Source: CAD feature listing. Evaluate the final solid. Frame: model axes, mm. A direction names the side the tool comes from. Give positions to 0.01 mm unless a question says otherwise; leave off trailing zeros. Order: outer loops, then holes, each group sorted by start corner. A loop starts at its lowest first (then second) coordinate and runs counter-clockwise, first axis right, second up. Notation, with made-up numbers: M 62,34 L 87,34 A9 ccw 87,43 Z; hole C -32,37.5 d10. An arc over 180 degrees is marked long. Answer in a Markdown table with one row per item. Add a question column.
(1) Pin query (flat end, axial travel): P1, Ø1.5, axis at x = -9, y = 8.5, coming from the -Z side; P2, Ø2, axis at y = 17.5, z = -16.5, coming from the -X side; P3, Ø1, axis at y = 12.5, z = -17.5, coming from the +X side. Return the tip coordinate at first contact, or that it passes through.
(2) Mould query, pull axis X, two halves, no side actions, for faces 4 (the face through (-25, 10, -30)), 5 (the face through (-20, 20, -5)), 6 (the face through (-22, 9.86, -24.54)). Classes: pulls with the +X half, pulls with the -X half, needs draft (parallel to the pull), parting line crosses it, or undercut.
(3) Section query C-C, the plane y = 8.5. Return loops of the section in (x, z).
(4) Section query A-A, the plane z = -9. Return loops of the section in (x, y).
(5) Section query D-D, the plane y = 18.5. Return loops of the section in (x, z), plus the area to 3 significant figures.
(6) Section query B-B, the plane x = -5. Return loops of the section in (y, z).
(7) Set-up query: faces 1 (the face through (-7.2, 9.9, -15)), 2 (the face through (-47.2, 9.9, -15)), 3 (the face through (-20, 0, -5)). Return all of +Z, -Z, +X, -X, +Y, -Y with unobstructed straight access to the full face (end or side cutting, diameter ignored); none if empty.
(8) Material intervals for line 1 along Y through (x, z) = (-5, -9.5); line 2 along Z through (x, y) = (-20.5, 18.75); line 3 along Z through (x, y) = (-5, 4), sorted ascending.
from build123d import *

# Parameters (mm, degrees)
BOSS_EXTRUDE1_DEPTH = 20
SKETCH3_R           = 10
CUT_EXTRUDE1_DEPTH  = 62.64414003
SKETCH4_R           = 2
CUT_EXTRUDE2_DEPTH  = 56.901699437


with BuildPart() as part:
    # Sketch2 → Boss-Extrude1 (new body)
    with BuildSketch(Plane(origin=(0, 0, 0), x_dir=(1, 0, 0), z_dir=(0, 1, 0))):
        with BuildLine():
            Line((-50, 0), (0, 0))
            Line((0, 0), (0, 15))
            Line((0, 15), (-10, 15))
            ThreePointArc((-10, 15), (-25, 30), (-40, 15))
            Line((-40, 15), (-50, 15))
            Line((-50, 15), (-50, 0))
        make_face()
    extrude(amount=BOSS_EXTRUDE1_DEPTH)

    # Sketch3 → Cut-Extrude1 (cut, through all)
    with BuildSketch(Plane(origin=(0, 0, 0), x_dir=(-1, 0, 0), z_dir=(0, -1, 0))):
        with Locations(Location((25, 15, 0), (0, 0, 90))):
            Circle(SKETCH3_R)
    extrude(amount=-CUT_EXTRUDE1_DEPTH, mode=Mode.SUBTRACT)

    # Sketch4 → Cut-Extrude2 (cut, through all)
    with BuildSketch(Plane(origin=(0, 0, -15), x_dir=(-1, 0, 0), z_dir=(0, 0, -1))):
        with Locations((45, 10)):
            Circle(SKETCH4_R)
        with Locations((5, 10)):
            Circle(SKETCH4_R)
    extrude(amount=-CUT_EXTRUDE2_DEPTH, mode=Mode.SUBTRACT)


solid = part.part
Values follow:
| question | item | result |
|---|---|---|
| 1 | P1 | stops at z = -15 |
| 1 | P2 | stops at x = -39.99 |
| 1 | P3 | stops at x = -10.13 |
| 2 | face 4 | parting line crosses it |
| 2 | face 5 | needs draft |
| 2 | face 6 | undercut |
| 3 | outline | M -50,-15 L -46.32,-15 L -46.32,0 L -50,0 Z; M -43.68,-15 L -40,-15 A15 ccw -10,-15 L -6.32,-15 L -6.32,0 L -43.68,0 Z; M -3.68,-15 L 0,-15 L 0,0 L -3.68,0 Z; hole C -25,-15 d20 |
| 4 | outline | M -50,0 L -33,0 L -33,20 L -50,20 Z; M -17,0 L 0,0 L 0,20 L -17,20 Z; hole C -45,10 d4; hole C -5,10 d4 |
| 5 | outline | M -50,-15 L -40,-15 A15 ccw -10,-15 L 0,-15 L 0,0 L -50,0 Z; hole C -25,-15 d20 |
| 5 | area | 789 mm² |
| 6 | outline | M 0,-15 L 8,-15 L 8,0 L 0,0 Z; M 12,-15 L 20,-15 L 20,0 L 12,0 Z |
| 7 | face 1 | -Z, +X, +Y, -Y |
| 7 | face 2 | -Z, -X, +Y, -Y |
| 7 | face 3 | +Z, -Z, +X, -X, -Y |
| 8 | line 1 | y = 0 to 8, 12 to 20 |
| 8 | line 2 | z = -29.31 to -23.93, -6.07 to 0 |
| 8 | line 3 | z = -15 to 0 |
